from build123d import *

# Parameters (mm, degrees)
BOSS_EXTRUDE1_DEPTH     = 38.1
CUT_EXTRUDE_THIN1_DEPTH = 30.48


with BuildPart() as part:
    # Sketch1 → Boss-Extrude1 (new body)
    with BuildSketch(Plane(origin=(0, 0, 0), x_dir=(1, 0, 0), z_dir=(0, 1, 0))):
        Polygon((-0.111992667, 54.937923296), (-38.926168882, 38.767787333), (-54.937923296, -0.111992667), (-38.767787333, -38.926168882), (0.111992667, -54.937923296), (38.926168882, -38.767787333), (54.937923296, 0.111992667), (38.767787333, 38.926168882), align=None)
    extrude(amount=BOSS_EXTRUDE1_DEPTH)

    # Sketch2 → Cut-Extrude-Thin1 (cut)
    with BuildSketch(Plane(origin=(0, 38.1, 0), x_dir=(1, 0, 0), z_dir=(0, 1, 0))):
        Polygon((24.950943415, -44.589920325), (17.176445042, -9.856652985), (-5.097897691, -19.136230336), (14.087218134, -49.115790304), (11.947790374, -50.484895435), (-8.86896141, -17.955664748), (18.993913528, -6.347883261), (27.429609427, -44.035109726), align=None)
        Polygon((-44.589920325, -24.950943415), (-9.856652985, -17.176445042), (-19.136230336, 5.097897691), (-49.115790304, -14.087218134), (-50.484895435, -11.947790374), (-17.955664748, 8.86896141), (-6.347883261, -18.993913528), (-44.035109726, -27.429609427), align=None)
        Polygon((-24.950943415, 44.589920325), (-17.176445042, 9.856652985), (5.097897691, 19.136230336), (-14.087218134, 49.115790304), (-11.947790374, 50.484895435), (8.86896141, 17.955664748), (-18.993913528, 6.347883261), (-27.429609427, 44.035109726), align=None)
        Polygon((44.589920325, 24.950943415), (9.856652985, 17.176445042), (19.136230336, -5.097897691), (49.115790304, 14.087218134), (50.484895435, 11.947790374), (17.955664748, -8.86896141), (6.347883261, 18.993913528), (44.035109726, 27.429609427), align=None)
    extrude(amount=-CUT_EXTRUDE_THIN1_DEPTH, mode=Mode.SUBTRACT)


solid = part.part
Verification items for the finished model (mm, model axes). A direction names the side the tool comes from. Coordinates: 2 decimals unless noted, no trailing zeros. Order: outer loops, then holes, each group sorted by start corner. A loop starts at its lowest first (then second) coordinate and runs counter-clockwise, first axis right, second up. Notation, with made-up numbers: (27, -15.5) -> (69, -15.5) arc R18 cw to (69, 15.5) -> close; hole circle Ø7 at (10, 57). An arc over 180 degrees is marked (long way). Put each result on its own line as item: value. Start each with the question number.
1. Material ranges on L1, parallel to Z at x = 29.5, y = 19; L2, parallel to Z at x = 12, y = 33.5; L3, parallel to Z at x = 41.5, y = 14, recorded low to high. Write a range as [from, to].
2. Cross-section at B-B, the plane z = 2.5. Record the boundary of the cut face in (x, y).
3. Mould release check, pull along X, two halves, no side actions. Record for faces 1 (the flat face through (19.6, 18.78, -46.82)), 2 (the flat face through (-4.892, 23.073, -12.223)), 3 (the flat face through (-46.966, 18.783, 19.247)): released by +X, released by -X, zero draft, split by the parting line, or undercut.
4. Access from +Z, -Z, +X, -X, +Y, -Y to the whole of each face (thin tool, end or side, straight path). Record for faces 4 (the flat face through (21.12, 23.07, 27.47)), 5 (the flat face through (-46.82, 18.78, -19.6)).
5. Cross-section at A-A, the plane y = 31.5. Count the separate pieces of the cut face and the enclosed holes in it, then the cut area to 3 significant figures.
6. Cross-section at C-C, the plane x = 21. Record the boundary of the cut face in (y, z).
7. Go/stop test with flat-tipped pins: pin 1 Ø5 at (x, y) = (11, 17) entering from -Z; pin 2 Ø1 at (x, y) = (39.5, 34) entering from -Z; pin 3 Ø2 at (x, y) = (42.5, 30.5) entering from -Z. Record where each tip stops, or that it passes through.
Computed:
1. L1: [-42.74, -24.18], [-21.57, -1.53], [1.48, 42.69]
1. L2: [-49.95, -20.26], [-17.66, -12.03], [-5.43, 9.26], [12.01, 45.85]
1. L3: [-32.37, -26.86], [-24.26, -9.21], [-6.2, 32.52]
2. outline: (-53.94, 0) -> (53.86, 0) -> (53.86, 38.1) -> (27.91, 38.1) -> (27.91, 7.62) -> (23.2, 7.62) -> (23.2, 38.1) -> (18.05, 38.1) -> (18.05, 7.62) -> (15.3, 7.62) -> (15.3, 38.1) -> (-13.22, 38.1) -> (-13.22, 7.62) -> (-15.97, 7.62) -> (-15.97, 38.1) -> (-31.01, 38.1) -> (-31.01, 7.62) -> (-35.72, 7.62) -> (-35.72, 38.1) -> (-53.94, 38.1) -> close
3. face 1: released by +X
3. face 2: undercut
3. face 3: released by -X
4. face 4: +Y
4. face 5: -Z, -X, +Y, -Y
5. separate pieces: 9
5. enclosed holes: 0
5. area: 7,520 mm2
6. outline: (0, -46.24) -> (38.1, -46.24) -> (38.1, -22.27) -> (7.62, -22.27) -> (7.62, -19.67) -> (38.1, -19.67) -> (38.1, 3.91) -> (7.62, 3.91) -> (7.62, 6.92) -> (38.1, 6.92) -> (38.1, 15.31) -> (7.62, 15.31) -> (7.62, 26.94) -> (38.1, 26.94) -> (38.1, 46.24) -> (0, 46.24) -> close
7. pin 1: z = -51.39
7. pin 2: z = -38.37
7. pin 3: z = -32.37
